Read the model definition and answer for the solid it produces. Units are mm, in the model's axes. Face numbers are marked on the shaded views. A direction names the side the tool comes from. Coordinates: 2 decimals unless noted, no trailing zeros. Order: outer loops, then holes, each group sorted by start corner. A loop starts at its lowest first (then second) coordinate and runs counter-clockwise, first axis right, second up. Notation, with made-up numbers: M 37,50 L 86,50 A35 cw 86,84 Z; hole C 6.5,89.5 d1. An arc over 180 degrees is marked long. Write each question's results on one line, items separated by ' | '.
Autodesk Inventor part; units mm, degrees
ref_plane "YZ Plane" through (0, 0, 0) normal (1, 0, 0) x (0, 1, 0)
ref_plane "XZ Plane" through (0, 0, 0) normal (0, 1, 0) x (-1, 0, 0)
ref_plane "XY Plane" through (0, 0, 0) normal (0, 0, 1) x (1, 0, 0)
sketch "Boceto1" plane through (0, 0, 0) normal (0, 1, 0) x (-1, 0, 0)
  circle A0 centre (0, 0) radius 8
  dimension "d0" = 16
extrude "Extrusión1" add sketch "Boceto1" along normal blind 46
sketch "Boceto2" plane through (0, 46, 0) normal (0, 1, 0) x (1, 0, 0)
  line L0 (0, 11.547) -> (10, 5.7735)
  line L1 (10, 5.7735) -> (10, -5.7735)
  line L2 (10, -5.7735) -> (0, -11.547)
  line L3 (0, -11.547) -> (-10, -5.7735)
  line L4 (-10, -5.7735) -> (-10, 5.7735)
  line L5 (-10, 5.7735) -> (0, 11.547)
  point P0 (0, 0)
  point P1 (0, 0)
  point P2 (-10, 0)
  dimension "d3" = 10
extrude "Extrusión2" add sketch "Boceto2" along normal blind 4
sketch "Boceto3" plane through (0, 0, 0) normal (0, -1, 0) x (1, 0, 0)
  circle A0 centre (0, 0) radius 8
  circle A1 centre (0, 0) radius 6
  dimension "d6" = 2
extrude "Extrusión3" cut sketch "Boceto3" against normal through all contours A1
sketch "Boceto4" plane through (0, 0, 0) normal (0, 0, 1) x (1, 0, 0)
  line L0 (-6, 0) -> (-6, 50)
  line L1 (6, 0) -> (6, 50)
  line L2 (-6, 0) -> (-6.5, 0)
  line L3 (-8, 0) -> (8, 0)
  line L4 (-6.5, 4) -> (-6.5, 0)
  line L5 (-6.5, 4) -> (-6, 4)
  line L6 (-6.5, 0) -> (-6, 0)
  line L7 (0, -14.3469) -> (0, 54.7161)
  line L8 (-6.5, 50) -> (-6.5, 46)
  line L9 (-6.5, 46) -> (-6, 46)
  line L10 (-10, 50) -> (0, 50)
  point P0 (0, 0)
  dimension "d9" = 0.5
  dimension "d10" = 4
  dimension "d11" = 0.5
  dimension "d12" = 4
revolve "Revolución1" cut sketch "Boceto4" angle 360 about axis through (0, -14.3469, 0) along (0, 1, 0) contours L2 L4 L5 L0 | L9 L8 L10 L0
properties part number "steering_stand_off_bush"
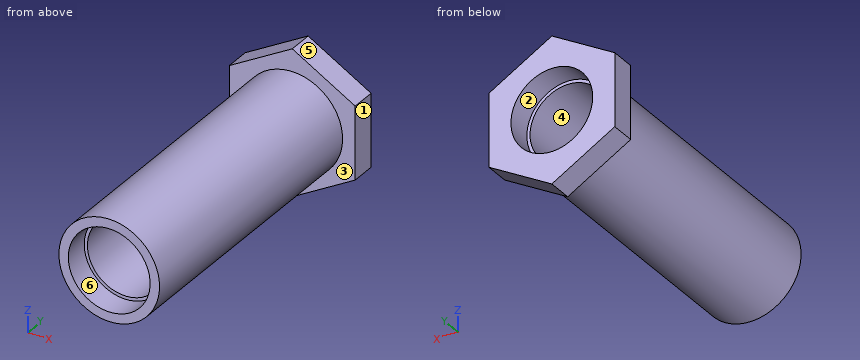
(1) Straight lines are drawn through the part: line 1 (Z direction, x = 0, y = 36); line 2 (Z direction, x = 0, y = 47); line 3 (Y direction, x = 3.25, z = 7.5). For each, find the intervals that lie inside material, in ascending order.
Conclusion:
line 1: -8 to -6, 6 to 8 | line 2: -11.55 to -6.5, 6.5 to 11.55 | line 3: 46 to 50
(2) The mould has two halves that part along X. Classify the marked faces 1, 2, 3 and 4: pulls with the +X half, pulls with the -X half, needs draft (parallel to the pull), parting line crosses it, or undercut.
Conclusion:
face 1: pulls with the +X half | face 2: undercut | face 3: needs draft | face 4: undercut
(3) The part is cut by section B-B, the plane x = 5.25. Write down the section's boundary in (y, z), then the cut area to 3 significant figures.
Conclusion:
outline: M 0,-6.04 L 46,-6.04 L 46,-8.52 L 50,-8.52 L 50,-3.83 L 46,-3.83 L 46,-2.9 L 4,-2.9 L 4,-3.83 L 0,-3.83 Z; M 0,3.83 L 4,3.83 L 4,2.9 L 46,2.9 L 46,3.83 L 50,3.83 L 50,8.52 L 46,8.52 L 46,6.04 L 0,6.04 Z | area: 318 mm²
(4) Given pin 1 (4 mm diameter, centred on y = 13, z = -8.5, fed in from +X); pin 2 (5 mm diameter, centred on y = 40.5, z = -7, fed in from -X); pin 3 (10.5 mm diameter, centred on x = -2.5, z = -0.5, fed in from +Y); pin 4 (2 mm diameter, centred on x = -1, z = 5, fed in from +Y), each flat-ended and moving along its own axis, determine where each tip first touches the part or whether it passes through.
Conclusion:
pin 1: x = 4.66 | pin 2: x = -6.61 | pin 3: y = 50 | pin 4: y = 46
(5) The part is cut by section D-D, the plane x = -7. Write down the section's boundary in (y, z).
Conclusion:
outline: M 0,-3.87 L 46,-3.87 L 46,-7.51 L 50,-7.51 L 50,7.51 L 46,7.51 L 46,3.87 L 0,3.87 Z
(6) The part is cut by section C-C, the plane y = 9.5. Write down the section's boundary in (x, z).
Conclusion:
outline: C 0,0 d16; hole C 0,0 d12
(7) For the marked faces 5 and 6, determine the directions among +Z, -Z, +X, -X, +Y, -Y from which every point of the face is accessible in a straight line to the end or side of a thin tool.
Conclusion:
face 5: +Z, +X, +Y, -Y | face 6: -Y
(8) The part is cut by section A-A, the plane z = 0. Write down the section's boundary in (x, y), then the cut area to 3 significant figures.
Conclusion:
outline: M -10,46 L -8,46 L -8,0 L -6.5,0 L -6.5,4 L -6,4 L -6,46 L -6.5,46 L -6.5,50 L -10,50 Z; M 6,4 L 6.5,4 L 6.5,0 L 8,0 L 8,46 L 10,46 L 10,50 L 6.5,50 L 6.5,46 L 6,46 Z | area: 208 mm²
